Geometry check sheet. Reference: the model listing, model coordinates, mm. Coordinates: 2 decimals unless noted, no trailing zeros. Write each loop counter-clockwise with the first axis right and the second up, starting at its lowest first coordinate (ties: lowest second). Pieces come first, ordered by that corner, then holes. Notation, with made-up numbers: M 5,32 L 63,32 A14 cw 63,50 Z; hole C 4,58.5 d2. An arc over 180 degrees is marked long. Write item = value, one per line. Start each with the question number.
```python
from build123d import *

# Parameters (mm, degrees)
CUT_EXTRUDE1_DEPTH  = 36.707142143
BOSS_EXTRUDE1_START = 5
BOSS_EXTRUDE1_DEPTH = 5
SKETCH7_R           = 0.75
CUT_EXTRUDE2_DEPTH  = 3


with BuildPart() as part:
    # Sketch4 → Revolve1 (revolve)
    with BuildSketch(Plane(origin=(0, 0, 0), x_dir=(1, 0, 0), z_dir=(0, 1, 0))):
        Polygon((0, 0), (0, 25), (2.5, 24), (5, 25), (5, 0), align=None)
    revolve(axis=Axis((5, 0, 0), (-1, 0, 0)))

    # Sketch5 → Cut-Extrude1 (cut, through all)
    with BuildSketch(Plane.ZY):
        Polygon((-15.722431864, 6.767949192), (-4.330127019, 2.5), (-13.722431864, 10.232050808), align=None)
        Polygon((-12.459478251, 11.737180314), (-3.213938048, 3.830222216), (-9.395300478, 14.308330752), align=None)
        Polygon((-7.693727678, 15.290734267), (-1.710100717, 4.698463104), (-3.934957195, 16.65881484), align=None)
        Polygon((0, 5), (2, 17), (-2, 17), align=None)
        Polygon((3.934957195, 16.65881484), (1.710100717, 4.698463104), (7.693727678, 15.290734267), align=None)
        Polygon((9.395300478, 14.308330752), (3.213938048, 3.830222216), (12.459478251, 11.737180314), align=None)
        Polygon((13.722431864, 10.232050808), (4.330127019, 2.5), (15.722431864, 6.767949192), align=None)
        Polygon((16.394435446, 4.921634526), (4.924038765, 0.868240888), (17.089028157, 0.982403514), align=None)
        Polygon((17.089028157, -0.982403514), (4.924038765, -0.868240888), (16.394435446, -4.921634526), align=None)
        Polygon((15.722431864, -6.767949192), (4.330127019, -2.5), (13.722431864, -10.232050808), align=None)
        Polygon((12.459478251, -11.737180314), (3.213938048, -3.830222216), (9.395300478, -14.308330752), align=None)
        Polygon((7.693727678, -15.290734267), (1.710100717, -4.698463104), (3.934957195, -16.65881484), align=None)
        Polygon((2, -17), (0, -5), (-2, -17), align=None)
        Polygon((-3.934957195, -16.65881484), (-1.710100717, -4.698463104), (-7.693727678, -15.290734267), align=None)
        Polygon((-9.395300478, -14.308330752), (-3.213938048, -3.830222216), (-12.459478251, -11.737180314), align=None)
        Polygon((-13.722431864, -10.232050808), (-4.330127019, -2.5), (-15.722431864, -6.767949192), align=None)
        Polygon((-16.394435446, -4.921634526), (-4.924038765, -0.868240888), (-17.089028157, -0.982403514), align=None)
        with BuildLine():
            ThreePointArc((-1.322875656, 1.5), (0, -2), (1.322875656, 1.5))
            Line((1.322875656, 1.5), (-1.322875656, 1.5))
        make_face()
        Polygon((-16.394435446, 4.921634526), (-17.089028157, 0.982403514), (-4.924038765, 0.868240888), align=None)
    extrude(amount=-CUT_EXTRUDE1_DEPTH, mode=Mode.SUBTRACT)

    # Sketch6 → Boss-Extrude1 (add)
    with BuildSketch(Plane.ZY.offset(BOSS_EXTRUDE1_START)):
        with BuildLine():
            Line((-3.570714214, 3.5), (3.570714214, 3.5))
            ThreePointArc((3.570714214, 3.5), (0, -5), (-3.570714214, 3.5))
        make_face()
        with BuildLine():
            Line((-1.322875656, 1.5), (1.322875656, 1.5))
            ThreePointArc((1.322875656, 1.5), (0, -2), (-1.322875656, 1.5))
        make_face(mode=Mode.SUBTRACT)
    extrude(amount=-BOSS_EXTRUDE1_DEPTH)

    # Sketch7 → Cut-Extrude2 (cut)
    with BuildSketch(Plane(origin=(0, 3.5, 0), x_dir=(1, 0, 0), z_dir=(0, 1, 0))):
        with Locations(Location((-3, 0, 0), (0, 0, 270))):
            Circle(SKETCH7_R)
    extrude(amount=-CUT_EXTRUDE2_DEPTH, mode=Mode.SUBTRACT)


solid = part.part
```
Q1. Cross-section at C-C on y = -12.5. Count the separate pieces of the cut face and the enclosed holes in it, and give its area (3 significant figures).
Q2. Cross-section at A-A on y = 0. Enter the section's corners in (x, z), and give its area (3 significant figures).
Q3. Gauge pin test, flat ends, axial feed: pin 1 (1 mm diameter, centred on x = 3, y = 15.5, fed in from -Z); pin 2 (1.5 mm diameter, centred on x = -1.5, z = 1.5, fed in from +Y); pin 3 (2.5 mm diameter, centred on y = 0, z = 0, fed in from -X); pin 4 (2 mm diameter, centred on x = 3.5, z = 1, fed in from +Y). Record the tip position at first contact, or that the pin passes through.
Q4. Draft check along Y on faces 1 (the face through (-3.665, 2.514, 0.346)), 2 (the face through (2.465, 10.762, 2.838)). Enter one of: pulls with the +Y half, pulls with the -Y half, needs draft (parallel to the pull), parting line crosses it, or undercut.
Q5. Scan lines: L1, parallel to X at y = 2.2, z = 0; L2, parallel to Z at x = 1, y = 11; L3, parallel to X at y = 3, z = 8. Record each from-to range of solid material in increasing order.
Q6. Cross-section at B-B on x = -3. Enter the section's corners in (y, z).
Values found:
q1.separate_pieces = 6
q1.enclosed_holes = 0
q1.area = 136 mm²
q2.outline = M -5,-5 L 0,-5 L 0,-25 L 2.5,-24 L 5,-25 L 5,-2 L -5,-2 Z; M -5,2 L 5,2 L 5,25 L 2.5,24 L 0,25 L 0,5 L -5,5 Z
q2.area = 255 mm²
q3.pin_1 = -19.07
q3.pin_2 = 3.5
q3.pin_3 = through
q3.pin_4 = 24.78
q4.face_1 = needs draft
q4.face_2 = undercut
q5.L1 = -5 to -3.75, -2.25 to 5
q5.L2 = -22 to -11.6, -7.44 to -5.27, -2.88 to -1, 1 to 2.88, 5.27 to 7.44, 11.6 to 22
q5.L3 = 0 to 5
q6.outline = M 1.5,-1.32 A2 cw long 1.5,1.32 L 1.5,0.75 L 3.5,0.75 L 3.5,3.57 A5 ccw long 3.5,-3.57 L 3.5,-0.75 L 1.5,-0.75 Z
